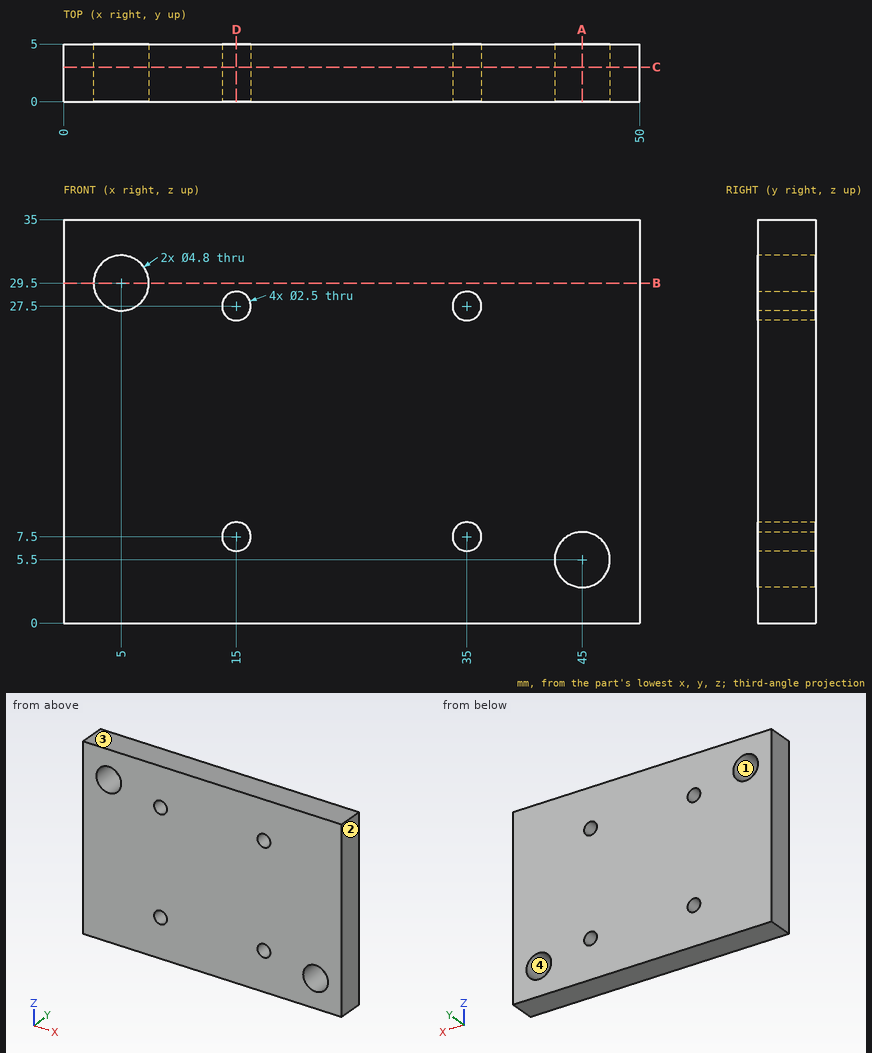
For this review, use the dimensioned drawing (mm, ordinates from the lowest corner) and the shaded views. Coordinates: 2 decimals unless noted, no trailing zeros. Write each loop counter-clockwise with the first axis right and the second up, starting at its lowest first coordinate (ties: lowest second). Pieces come first, ordered by that corner, then holes. Notation, with made-up numbers: (4, 62.5) - (32, 62.5) arc R22 cw to (32, 84.5) - close; hole circle Ø6 at (-12.75, -10.75). An arc over 180 degrees is marked (long way). Answer as a JSON object with one key per item and string values. Group by question number.
1. To check wall thickness, follow probe 1 along Z at (x, y) = (35, 2.35); probe 2 along X at (y, z) = (3.2, 5.5); probe 3 along X at (y, z) = (3.4, 27.5). State the ranges of each line that lie inside material, in increasing order.
2. Mouldability with a two-part tool opening along Z and no side actions: class the marked faces 1, 2, 3 and 4 as pulls with the +Z half, pulls with the -Z half, needs draft (parallel to the pull), parting line crosses it, or undercut.
3. Add section B-B (z = 29.5). Give the boundary of the cut face in (x, y), plus the area to 3 significant figures.
4. Add section C-C (y = 3). Give the boundary of the cut face in (x, z), plus the area to 3 significant figures.
5. Add section D-D (x = 15). Give the boundary of the cut face in (y, z).
6. Add section A-A (x = 45). Give the boundary of the cut face in (y, z), plus the area to 3 significant figures.
Findings:
{
 "1": {"probe 1": "0 to 6.25, 8.75 to 26.25, 28.75 to 35", "probe 2": "0 to 42.6, 47.4 to 50", "probe 3": "0 to 3.67, 6.33 to 13.75, 16.25 to 33.75, 36.25 to 50"},
 "2": {"face 1": "undercut", "face 2": "needs draft", "face 3": "pulls with the +Z half", "face 4": "undercut"},
 "3": {"outline": "(0, 0) - (2.6, 0) - (2.6, 5) - (0, 5) - close; (7.4, 0) - (50, 0) - (50, 5) - (7.4, 5) - close", "area": "226 mm²"},
 "4": {"outline": "(0, 0) - (50, 0) - (50, 35) - (0, 35) - close; hole circle Ø4.8 at (5, 29.5); hole circle Ø2.5 at (15, 7.5); hole circle Ø2.5 at (15, 27.5); hole circle Ø2.5 at (35, 7.5); hole circle Ø2.5 at (35, 27.5); hole circle Ø4.8 at (45, 5.5)", "area": "1,690 mm²"},
 "5": {"outline": "(0, 0) - (5, 0) - (5, 6.25) - (0, 6.25) - close; (0, 8.75) - (5, 8.75) - (5, 26.25) - (0, 26.25) - close; (0, 28.75) - (5, 28.75) - (5, 35) - (0, 35) - close"},
 "6": {"outline": "(0, 0) - (5, 0) - (5, 3.1) - (0, 3.1) - close; (0, 7.9) - (5, 7.9) - (5, 35) - (0, 35) - close", "area": "151 mm²"}
}
